from build123d import *

# Parameters (mm, degrees)
BOSS_EXTRUDE5_START = -4.7625
BOSS_EXTRUDE5_DEPTH = 9.525
SKETCH6_R           = 1.778
CUT_EXTRUDE3_DEPTH  = 504.733086563
CUT_EXTRUDE4_START  = 3.556
SKETCH7_R           = 3.048
SKETCH7_R_2         = 1.778
CUT_EXTRUDE4_DEPTH  = 505.502600354
CUT_EXTRUDE5_DEPTH  = 506.075936751


# Read off the part's stored shape, not the designer's step: Boss-Extrude5
with BuildPart() as part:
    # Boss-Extrude5 outline → Boss-Extrude5 (new body)
    with BuildSketch(Plane(origin=(0, 0, 4.097149242), x_dir=(-1, 0, 0), z_dir=(0, 0, -1)).offset(BOSS_EXTRUDE5_START)):
        with BuildLine():
            add(Edge.make_bspline(
                [(398.35171036, -68.196818162), (396.265786035, -68.16801087), (352.35609282, -67.485074441), (308.459309619, -65.190615284), (266.801551376, -61.551589611)],
                knots=[0.388247103, 0.388247103, 0.388247103, 0.388247103, 0.401472843, 0.666666775, 0.666666775, 0.666666775, 0.666666775], degree=3))
            ThreePointArc((398.35171036, -68.196818162), (445.202941044, -75.692238551), (487.961522574, -96.257326662))
            ThreePointArc((487.961522574, -96.257326662), (494.102034598, -94.922101367), (492.499924864, -88.845757162))
            ThreePointArc((492.499924864, -88.845757162), (472.347982204, -65.669309605), (471.824439099, -34.961421092))
            ThreePointArc((471.824439099, -34.961421092), (471.408544547, -32.082865726), (468.823110549, -30.750731982))
            Line((468.823110549, -30.750731982), (459.298110549, -30.750731982))
            ThreePointArc((459.298110549, -30.750731982), (456.664489609, -32.15241144), (456.356218194, -35.119840174))
            ThreePointArc((456.356218194, -35.119840174), (459.13228847, -45.417631787), (459.332762362, -56.081162557))
            ThreePointArc((459.332762362, -56.081162557), (457.466080229, -59.75328384), (453.620807302, -61.230731982))
            Line((453.620807302, -61.230731982), (423.379813153, -61.230732209))
            add(Edge.make_bspline(
                [(384.696694825, -60.817291125), (385.490946956, -60.834366335), (398.383584309, -61.102948796), (411.282715888, -61.232192999), (423.379813153, -61.230732209)],
                knots=[0.584578014, 0.584578014, 0.584578014, 0.584578014, 0.589634714, 0.666658831, 0.666658831, 0.666658831, 0.666658831], degree=3))
            ThreePointArc((384.696694825, -60.817291125), (381.405012252, -59.519394589), (379.749008052, -56.392517605))
            ThreePointArc((379.749008052, -56.392517605), (379.962938882, -45.344267983), (383.481055682, -34.868942675))
            ThreePointArc((383.481055682, -34.868942675), (383.390574332, -31.793909155), (380.736068027, -30.23904122))
            add(Edge.make_bspline(
                [(371.231646974, -29.984054972), (374.399550345, -30.077611409), (377.567706075, -30.162607104), (380.736068027, -30.23904122)],
                knots=[0.554089987, 0.554089987, 0.554089987, 0.554089987, 0.574612442, 0.574612442, 0.574612442, 0.574612442], degree=3))
            ThreePointArc((371.231646974, -29.984054972), (368.497590253, -31.39435755), (368.242362699, -34.460116724))
            ThreePointArc((368.242362699, -34.460116724), (371.193755258, -45.109007009), (370.814996268, -56.152834373))
            ThreePointArc((370.814996268, -56.152834373), (368.993717887, -59.186422189), (365.637179769, -60.305958601))
            add(Edge.make_bspline(
                [(301.916083239, -57.118764264), (304.793492849, -57.314159562), (316.447125042, -58.077219349), (336.889920622, -59.214945623), (355.259103136, -59.965814652), (364.843153704, -60.280423032), (365.637179769, -60.305958601)],
                knots=[0.408750601, 0.408750601, 0.408750601, 0.408750601, 0.427107919, 0.483087827, 0.539067736, 0.544124431, 0.544124431, 0.544124431, 0.544124431], degree=3))
            ThreePointArc((301.916083239, -57.118764264), (297.703900514, -55.115863145), (295.996304567, -50.7755622))
            ThreePointArc((295.996304567, -50.7755622), (297.395526272, -40.599539879), (301.466201974, -31.168800195))
            ThreePointArc((301.466201974, -31.168800195), (301.565948035, -28.066269557), (298.971867926, -26.361454603))
            add(Edge.make_bspline(
                [(289.489598636, -25.664595471), (292.649719638, -25.90542225), (295.810491414, -26.137709697), (298.971867926, -26.361454603)],
                knots=[0.377389823, 0.377389823, 0.377389823, 0.377389823, 0.397912285, 0.397912285, 0.397912285, 0.397912285], degree=3))
            ThreePointArc((289.489598636, -25.664595471), (286.640803233, -27.018955044), (286.365734252, -30.161288915))
            ThreePointArc((286.365734252, -30.161288915), (289.309950073, -39.618561112), (289.709550194, -49.515465879))
            ThreePointArc((289.709550194, -49.515465879), (287.468803622, -53.805389908), (282.855937937, -55.270266537))
            Line((282.855937937, -55.270266537), (268.113256948, -54.036580381))
            add(Edge.make_bspline(
                [(268.113256948, -54.036580381), (262.634745624, -53.56111419), (251.663313863, -52.628696852), (229.81175043, -50.89541865), (191.471827261, -48.203857237), (136.679597141, -45.286916485), (81.835702382, -43.641470214), (43.402846546, -43.138474088), (21.480818831, -43.050269737), (10.476996172, -43.067138198), (4.980483945, -43.087244707)],
                knots=[-0.002434158, -0.002434158, -0.002434158, -0.002434158, 0.060213256, 0.12286067, 0.248155497, 0.498745152, 0.749334808, 0.874629635, 0.937277049, 0.999924463, 0.999924463, 0.999924463, 0.999924463], degree=3))
            Line((4.980483945, -43.087244707), (5.013364858, -50.687454907))
            add(Edge.make_bspline(
                [(266.801551376, -61.551589611), (261.350884009, -61.078554924), (250.433518448, -60.153958667), (228.701217873, -58.434486699), (190.548987698, -55.763104255), (136.042529388, -52.86929541), (81.4824687, -51.236835025), (43.240954482, -50.737883821), (21.43842692, -50.650632415), (10.483916541, -50.667450636), (5.013364858, -50.687454907)],
                knots=[4.0417e-05, 4.0417e-05, 4.0417e-05, 4.0417e-05, 0.062531963, 0.125023508, 0.2500066, 0.499972783, 0.749938966, 0.874922057, 0.937413603, 0.999905149, 0.999905149, 0.999905149, 0.999905149], degree=3))
        make_face()
    boss_extrude5 = extrude(amount=BOSS_EXTRUDE5_DEPTH)

    # Sketch6 → Cut-Extrude3 (cut, through all)
    with BuildSketch(Plane(origin=(0.32087569, -4.366204823, 0), x_dir=(0.9973104440526221, 0.07329309778936742, 0), z_dir=(-0.07329309778936742, 0.9973104440526221, 0))):
        with Locations(Location((-295.980145151, -4.097149242, 0), (0, 0, 180))):
            Circle(SKETCH6_R)
    cut_extrude3 = extrude(amount=-CUT_EXTRUDE3_DEPTH, mode=Mode.SUBTRACT)

    # Sketch7 → Cut-Extrude4 (cut)
    with BuildSketch(Plane(origin=(3.065947832, -41.718823267, 0), x_dir=(-0.9946544730103679, -0.07309790847145088, 0.07293267510222654), z_dir=(-0.07329309778936742, 0.9973104440526221, 0)).offset(CUT_EXTRUDE4_START)):
        with Locations(Location((295.490726509, -17.500385777, 0), (0, 0, 355.817552062))):
            Circle(SKETCH7_R)
        with Locations(Location((295.490726509, -17.500385777, 0), (0, 0, 355.817552062))):
            Circle(SKETCH7_R_2, mode=Mode.SUBTRACT)
    cut_extrude4 = extrude(amount=-CUT_EXTRUDE4_DEPTH, mode=Mode.SUBTRACT)

    # Mirror4: Boss-Extrude5, Cut-Extrude3, Cut-Extrude4 across plane
    add(boss_extrude5.mirror(Plane(origin=(-4.793985166, 0.020740296, 8.859649242), x_dir=(0, 0, 1), z_dir=(-0.9999906416249494, 0.004326275825933448, 0))))
    add(cut_extrude3.mirror(Plane(origin=(-4.793985166, 0.020740296, 8.859649242), x_dir=(0, 0, 1), z_dir=(-0.9999906416249494, 0.004326275825933448, 0))), mode=Mode.SUBTRACT)
    add(cut_extrude4.mirror(Plane(origin=(-4.793985166, 0.020740296, 8.859649242), x_dir=(0, 0, 1), z_dir=(-0.9999906416249494, 0.004326275825933448, 0))), mode=Mode.SUBTRACT)

    # Sketch9 → Cut-Extrude5 (cut, through all)
    with BuildSketch(Plane(origin=(0, 0, -0.665350758), x_dir=(-1, 0, 0), z_dir=(0, 0, -1))):
        Polygon((268.113256948, -54.036580381), (282.855937937, -55.270266537), (282.538222795, -59.066996326), (267.795541806, -57.83331017), (267.467078991, -61.609602167), (-501.730233012, -147.179806135), (-501.730233012, -16.830462442), (271.226711866, -16.830462442), align=None)
    extrude(amount=-CUT_EXTRUDE5_DEPTH, mode=Mode.SUBTRACT)


solid = part.part
Here's how the part is built. I have some questions about the finished solid (model axes, mm). A direction names the side the tool comes from. Round coordinates to 2 decimals unless told otherwise and drop trailing zeros. Loops run counter-clockwise (first coordinate to the right, second up) from the corner with the lowest first, then second, coordinate; pieces in that order, holes last.
1. We'd pull the mould along Z, two halves only. Please class faces 1 (the face through (-295.144, -61.911, 5.013)), 2 (the face through (-294.36, -60.01, 4.14)), 3 (the face through (-464, -30.751, 4)), 4 (the face through (-388.8, -61.2, 8.86)): +Z half, -Z half, draft (parallel to the pull), parting line (faces both ways), or undercut.
Answer list:
face 1: undercut
face 2: undercut
face 3: draft
face 4: +Z half
2. If I drill on line 1 along X through (y, z) = (-45.5, 1.75); line 2 along X through (y, z) = (-43, 0); line 3 along X through (y, z) = (-37.5, 4.75), over which ranges is the centre line in solid material (lowest first)?
Answer list:
line 1: x = -469.56 to -459.14, -379.94 to -371.24, -296.37 to -289.86
line 2: x = -469.86 to -458.72, -380.45 to -370.88, -296.81 to -289.74
line 3: x = -471.03 to -457.24, -382.25 to -369.45, -298.41 to -295.68, -292.36 to -288.88
3. If we section it at A-A on y = -47.5: Count the separate pieces of the cut face and the enclosed holes in it, plus the area to 3 significant figures.
Answer list:
separate pieces: 3
enclosed holes: 1
area: 224 mm2
4. If we section it at C-C on y = -72.5: Write out the boundary of the cut face in (x, z), plus the area to 3 significant figures.
Answer list:
outline: (-475.66, -0.67) - (-433.51, -0.67) - (-433.51, 8.86) - (-475.66, 8.86) - close
area: 401 mm2
5. If we section it at B-B on x = -444: Write out the boundary of the cut face in (y, z), plus the area to 3 significant figures.
Answer list:
outline: (-75.32, -0.67) - (-61.23, -0.67) - (-61.23, 8.86) - (-75.32, 8.86) - close
area: 134 mm2
6. Which directions (+Z, -Z, +X, -X, +Y, -Y) give clear straight access to the entire face, cutting with the end or side of a thin tool? Please do faces 5 (the face through (-289.286, -39.482, 4.164)), 6 (the face through (-439, -61.231, 4)), 7 (the face through (-297.75, -55.165, 4.164)).
Answer list:
face 5: +Z, -Z, +X
face 6: +Z, -Z, +Y
face 7: +Z, -Z
7. For P1, Ø1.5, axis at x = -337.5, y = -68, coming from the -Z side, with a flat end and sliding along its axis, tell me the tip position at first contact or that it passes through.
Answer list:
P1: passes through
